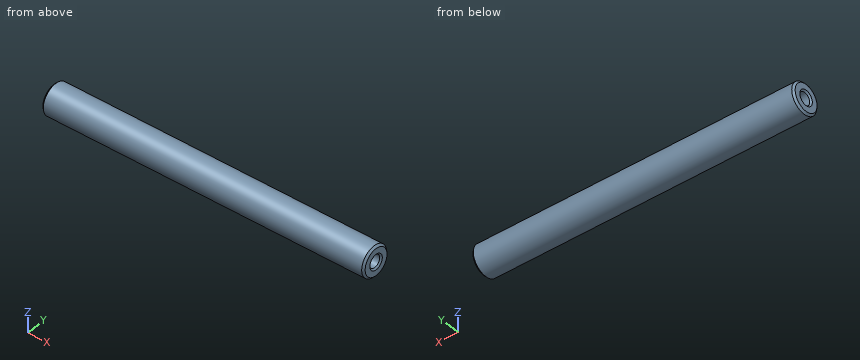
Autodesk Inventor part; units mm, degrees
ref_plane "YZ Plane" through (0, 0, 0) normal (1, 0, 0) x (0, 1, 0)
ref_plane "XZ Plane" through (0, 0, 0) normal (0, 1, 0) x (-1, 0, 0)
ref_plane "XY Plane" through (0, 0, 0) normal (0, 0, 1) x (1, 0, 0)
sketch "Sketch_1" plane through (0, 0, 0) normal (0, 0, 1) x (1, 0, 0)
  line L0 (86, 0) -> (0, 0)
  line L1 (0, 0) -> (0, 3.5)
  line L2 (0, 3.5) -> (0.5, 4)
  line L3 (0.5, 4) -> (85.5, 4)
  line L4 (85.5, 4) -> (86, 3.5)
  line L5 (86, 3.5) -> (86, 0)
  line L6 (86, 0) -> (0, 0)
revolve "Revolution1" add sketch "Sketch_1" angle 360 about axis through (86, 0, 0) along (1, 0, 0)
sketch "Sketch2" plane through (0, 0, 0) normal (-1, 0, 0) x (0, 0, 1)
  point P0 (0, 0)
hole "Hole1" at (0, 0, 0) direction (1, 0, 0) diameter 3.242 depth 9.0641 tip angle 120 countersink diameter 4 countersink angle 90
sketch "Sketch3" plane through (86, 0, 0) normal (1, 0, 0) x (0, 0, -1)
  point P0 (0, 0)
hole "Hole2" at (86, 0, 0) direction (-1, 0, 0) diameter 3.242 depth 9.0241 tip angle 120 countersink diameter 4 countersink angle 90
properties part number "RDOB8-86-WMC4"
Can you work these out from the model? Positions are in its coordinate system, mm. Coordinates: 2 decimals unless noted, no trailing zeros. Write each loop counter-clockwise with the first axis right and the second up, starting at its lowest first coordinate (ties: lowest second). Pieces come first, ordered by that corner, then holes. Notation, with made-up numbers: M 74.5,16 L 94.5,16 A35 ccw 94.5,52 Z; hole C -17.75,-6.5 d4. An arc over 180 degrees is marked long. Use one line per item in the form item = value.
Q1. If we section it at A-A (x = 25): Write out the boundary of the cut face in (y, z), then the cut area to 3 significant figures.
Model answer:
outline = C 0,0 d8
area = 50.3 mm^2
Q2. I need wall thicknesses on line 1 along Z through (x, y) = (4.5, 0); line 2 along X through (y, z) = (3.5, -0.25); line 3 along Y through (x, z) = (39, 2.5). Which ranges of each line are inside material? Lowest first, please. Write a range as from..to.
Model answer:
line_1 = -4..-1.62, 1.62..4
line_2 = 0.01..85.99
line_3 = -3.12..3.12
Q3. For P1, Ø1, axis at x = 71, z = -1, coming from the -Y side; P2, Ø1.5, axis at x = 11.5, y = -1, coming from the +Z side; P3, Ø2.5, axis at y = 0, z = 0, coming from the -X side, each with a flat end and sliding along its axis, tell me the tip position at first contact or that it passes through.
Model answer:
P1 = -3.97
P2 = 3.99
P3 = 9.28
